```python
from build123d import *

# Parameters (mm, degrees)
SKETCH1_W                = 25
SKETCH1_H                = 6.75
BOSS_EXTRUDE1_DEPTH      = 6.5
BOSS_EXTRUDE4_DEPTH      = 6.5
BOSS_EXTRUDE3_DEPTH      = 6
BOSS_EXTRUDE3_DEPTH_BACK = 4.95
SKETCH4_W                = 2.3
SKETCH4_H                = 4.5
CUT_EXTRUDE1_DEPTH       = 23
SKETCH6_R                = 2.55
CUT_EXTRUDE2_DEPTH       = 10
BOSS_EXTRUDE5_DEPTH      = 1.575
CUT_EXTRUDE3_DEPTH       = 3
SKETCH9_R                = 0.8
CUT_EXTRUDE4_DEPTH       = 10.95
BOSS_EXTRUDE6_DEPTH      = 0.25


with BuildPart() as part:
    # Sketch1 → Boss-Extrude1 (new body)
    with BuildSketch(Plane(origin=(0, 0, 0), x_dir=(1, 0, 0), z_dir=(0, 1, 0))):
        with Locations((12.5, -3.375)):
            Rectangle(SKETCH1_W, SKETCH1_H)
    extrude(amount=BOSS_EXTRUDE1_DEPTH)

    # Sketch5 → Boss-Extrude4 (add)
    with BuildSketch(Plane(origin=(0, 6.5, 0), x_dir=(1, 0, 0), z_dir=(0, 1, 0))):
        Polygon((-5.715767665, -3.375), (-2.857883832, -8.325), (2.857883832, -8.325), (5.715767665, -3.375), (2.857883832, 1.575), (-2.857883832, 1.575), align=None)
    extrude(amount=-BOSS_EXTRUDE4_DEPTH)

    # Sketch3 → Boss-Extrude3 (add, two sides)
    with BuildSketch(Plane.XY.offset(3.375)) as boss_extrude3_sk:
        Polygon((22.599882374, 14.546249674), (27.562613132, 15.155596391), (30, -4.695326641), (25.037269242, -5.304673359), align=None)
    extrude(amount=BOSS_EXTRUDE3_DEPTH)
    extrude(boss_extrude3_sk.sketch, amount=-BOSS_EXTRUDE3_DEPTH_BACK)

    # Sketch4 → Cut-Extrude1 (cut)
    with BuildSketch(Plane(origin=(-1.423871601, 11.596503591, 0), x_dir=(0.992546152, 0.121869343, 0), z_dir=(-0.121869343, 0.992546152, 0))):
        with Locations((28.054168174, -2.675)):
            Rectangle(SKETCH4_W, SKETCH4_H)
    extrude(amount=-CUT_EXTRUDE1_DEPTH, mode=Mode.SUBTRACT)

    # Sketch6 → Cut-Extrude2 (cut)
    with BuildSketch(Plane(origin=(0, 6.5, 0), x_dir=(1, 0, 0), z_dir=(0, 1, 0))):
        with Locations((0, -3.335615973)):
            Circle(SKETCH6_R)
    extrude(amount=-CUT_EXTRUDE2_DEPTH, mode=Mode.SUBTRACT)

    # Sketch7 → Boss-Extrude5 (add)
    with BuildSketch(Plane(origin=(0, 0, -1.575), x_dir=(-1, 0, 0), z_dir=(0, 0, -1))):
        Polygon((-2.857883832, 0), (-24.385937253, 0), (-25.037269242, -5.304673359), (-30, -4.695326641), (-27.562613132, 15.155596391), (-22.599882374, 14.546249674), (-23.587837607, 6.5), (-2.857883832, 6.5), align=None)
    extrude(amount=-BOSS_EXTRUDE5_DEPTH)

    # Sketch8 → Cut-Extrude3 (cut)
    with BuildSketch(Plane(origin=(0, 0, 0), x_dir=(-1, 0, 0), z_dir=(0, -1, 0))):
        Polygon((-4.67653718, -11.475), (4.67653718, -11.475), (9.353074361, -3.375), (4.67653718, 4.725), (-4.67653718, 4.725), (-9.353074361, -3.375), align=None)
    extrude(amount=-CUT_EXTRUDE3_DEPTH, mode=Mode.SUBTRACT)

    # Sketch9 → Cut-Extrude4 (cut)
    with BuildSketch(Plane(origin=(0, 0, -1.575), x_dir=(-1, 0, 0), z_dir=(0, 0, -1))):
        with Locations((-28.526885988, -3.36493756)):
            Circle(SKETCH9_R)
        with Locations((-27.917539271, 1.597793198)):
            Circle(SKETCH9_R)
        with Locations((-27.308192554, 6.560523956)):
            Circle(SKETCH9_R)
        with Locations((-26.698845837, 11.523254714)):
            Circle(SKETCH9_R)
    extrude(amount=-CUT_EXTRUDE4_DEPTH, mode=Mode.SUBTRACT)

    # Sketch10 → Boss-Extrude6 (add)
    with BuildSketch(Plane.XY.offset(6.75)):
        Polygon((11.311801843, 5.121255448), (13.555391587, 5.121255448), (13.555391587, 4.795233814), (12.011521395, 1.531511859), (11.454830689, 1.811960577), (12.744894792, 4.537922115), (11.311801843, 4.537922115), align=None)
        Polygon((14.542571074, 5.210999038), (15.125904407, 5.210999038), (14.980071074, 4.537922115), (15.523440465, 5.013983814), (15.798981331, 4.537922115), (15.081032613, 4.335999038), (15.798981331, 4.134075961), (15.488384375, 3.647497435), (14.961841907, 4.134075961), (15.125904407, 3.460999038), (14.542571074, 3.460999038), (14.719954888, 4.134075961), (14.18149335, 3.647497435), (13.869494151, 4.134075961), (14.587442869, 4.335999038), (13.869494151, 4.537922115), (14.18149335, 5.036419711), (14.719954888, 4.537922115), align=None)
    extrude(amount=BOSS_EXTRUDE6_DEPTH)


solid = part.part
```
Could you check a few things on this model? Use its own coordinates, in mm. A direction names the side the tool comes from. Coordinates: 2 decimals unless noted, no trailing zeros. Write each loop counter-clockwise with the first axis right and the second up, starting at its lowest first coordinate (ties: lowest second). Pieces come first, ordered by that corner, then holes. Notation, with made-up numbers: (-17.75, -13.75) - (16.25, -13.75) arc R10 ccw to (16.25, -6.75) - close; hole circle Ø10 at (-33.75, 30.5). An arc over 180 degrees is marked (long way). Use a Markdown table: item, result.
Q1. I'm going to push flat-ended pins straight in: pin 1 Ø1.4 at (x, y) = (28.53, -3.36) entering from -Z; pin 2 Ø6 at (y, z) = (12, 5) entering from -X; pin 3 Ø6 at (y, z) = (10, 4) entering from -X; pin 4 Ø1 at (y, z) = (7.5, 3.5) entering from -X. Where does each tip first touch, or does it pass through?
Geometry check:
| item | result |
|---|---|
| pin 1 | passes through |
| pin 2 | stops at x = 22.6 |
| pin 3 | stops at x = 22.79 |
| pin 4 | stops at x = 23.4 |
Q2. Thinking about a two-plate mould opening in X: for faces 1 (the flat face through (26, 5, 9.375)), 2 (the flat face through (8.39, 1.48, 5.04)), 3 (the cylindrical face through (28.717, 1.633, 7.119)), 4 (the flat face through (28.764, 5.369, -0.561)), which applies, +X half, -X half, draft (parallel to the pull), parting line (faces both ways), or undercut?
Geometry check:
| item | result |
|---|---|
| face 1 | draft |
| face 2 | -X half |
| face 3 | undercut |
| face 4 | +X half |
Q3. Imagine slicing it at A-A (x = 0). List the corners of the cut face in (y, z) for me (3 decimals), and give its area (3 significant figures).
Geometry check:
| item | result |
|---|---|
| outline | (3, -1.575) - (6.5, -1.575) - (6.5, 0.786) - (3, 0.786) - close; (3, 5.886) - (6.5, 5.886) - (6.5, 8.325) - (3, 8.325) - close |
| area | 16.8 mm2 |
Q4. Imagine slicing it at D-D (z = 4.25). List the corners of the cut face in (x, y) for me.
Geometry check:
| item | result |
|---|---|
| outline | (-5.21, 3) - (-2.38, 3) - (-2.38, 6.5) - (-5.21, 6.5) - close; (2.38, 3) - (8.85, 3) - (8.85, 0) - (24.39, 0) - (25.04, -5.3) - (27.72, -4.98) - (25.28, 14.88) - (22.6, 14.55) - (23.59, 6.5) - (2.38, 6.5) - close |
Q5. Please list where these lines run through material, in increasing order: L1, parallel to Y at x = 27, z = 6.25; L2, parallel to Y at x = 14, z = 0; L3, parallel to Z at x = 20, y = 2.75 (3 decimals).
Geometry check:
| item | result |
|---|---|
| L1 | y = -5.06 to 5.82, 7.3 to 10.78, 12.26 to 15.09 |
| L2 | y = 0 to 6.5 |
| L3 | z = -1.575 to 6.75 |
Q6. Imagine slicing it at C-C (x = 17.5). List the corners of the cut face in (y, z) for me (3 decimals), and give its area (3 significant figures).
Geometry check:
| item | result |
|---|---|
| outline | (0, -1.575) - (6.5, -1.575) - (6.5, 6.75) - (0, 6.75) - close |
| area | 54.1 mm2 |
Q7. Imagine slicing it at B-B (z = 2.75). List the corners of the cut face in (x, y) for me, and give its area (3 significant figures).
Geometry check:
| item | result |
|---|---|
| outline | (-5.35, 3) - (-2.48, 3) - (-2.48, 6.5) - (-5.35, 6.5) - close; (2.48, 3) - (8.99, 3) - (8.99, 0) - (24.39, 0) - (25.04, -5.3) - (27.72, -4.98) - (25.28, 14.88) - (22.6, 14.55) - (23.59, 6.5) - (2.48, 6.5) - close |
| area | 184 mm2 |
Q8. Which directions (+Z, -Z, +X, -X, +Y, -Y) give clear straight access to the entire face, cutting with the end or side of a thin tool? Please do faces 5 (the flat face through (3.306, 4.774, 7.549)), 6 (the flat face through (0, 5, 8.325)), 7 (the flat face through (28, 5, 4.925)).
Geometry check:
| item | result |
|---|---|
| face 5 | +Z, +Y, -Y |
| face 6 | +Z, -X, +Y, -Y |
| face 7 | +X, +Y |
